Geometry: final body of the model. Coordinates: model frame, mm. Face numbers are marked on the shaded views. A direction names the side the tool comes from. Give positions to 0.01 mm unless a question says otherwise; leave off trailing zeros. Write each loop counter-clockwise with the first axis right and the second up, starting at its lowest first coordinate (ties: lowest second). Pieces come first, ordered by that corner, then holes. Notation, with made-up numbers: (-23.5, -27) -> (-19.5, -27) arc R25 cw to (-19.5, 5) -> close; hole circle Ø1 at (45, 17). An arc over 180 degrees is marked (long way). Answer in a Markdown table with one row per item. Add a question column.
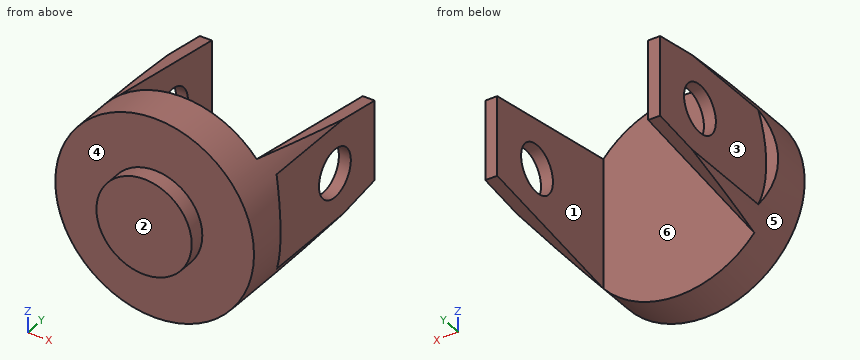
from build123d import *

# Parameters (mm, degrees)
SKETCH1_R               = 125
BOSS_EXTRUDE1_DEPTH     = 250
SKETCH3_W               = 190
SKETCH3_H               = 250
CUT_EXTRUDE1_DEPTH      = 200
CUT_EXTRUDE3_DEPTH      = 221
CUT_EXTRUDE3_DEPTH_BACK = 31
SKETCH8_R               = 30
CUT_EXTRUDE4_DEPTH      = 221
CUT_EXTRUDE4_DEPTH_BACK = 31
SKETCH6_R               = 125
CUT_EXTRUDE8_DEPTH      = 60
SKETCH7_R               = 125
CUT_EXTRUDE9_DEPTH      = 60
SKETCH9_R               = 59.95
BOSS_EXTRUDE2_DEPTH     = 20


with BuildPart() as part:
    # Sketch1 → Boss-Extrude1 (new body)
    with BuildSketch(Plane(origin=(0, 0, 0), x_dir=(1, 0, 0), z_dir=(0, 1, 0))):
        Circle(SKETCH1_R)
    extrude(amount=BOSS_EXTRUDE1_DEPTH)

    # Sketch3 → Cut-Extrude1 (cut)
    with BuildSketch(Plane(origin=(0, 250, 0), x_dir=(1, 0, 0), z_dir=(0, 1, 0))):
        Rectangle(SKETCH3_W, SKETCH3_H)
    extrude(amount=-CUT_EXTRUDE1_DEPTH, mode=Mode.SUBTRACT)

    # Sketch4 → Cut-Extrude3 (cut, two sides)
    with BuildSketch(Plane(origin=(-95, 0, 0), x_dir=(0, 0, -1), z_dir=(1, 0, 0))) as cut_extrude3_sk:
        Polygon((-81.240384046, 250), (-81.240384046, 50), (-50, 250), align=None)
        Polygon((50, 250), (81.240384046, 50), (81.240384046, 250), align=None)
    extrude(amount=CUT_EXTRUDE3_DEPTH, mode=Mode.SUBTRACT)
    extrude(cut_extrude3_sk.sketch, amount=-CUT_EXTRUDE3_DEPTH_BACK, mode=Mode.SUBTRACT)

    # Sketch8 → Cut-Extrude4 (cut, two sides)
    with BuildSketch(Plane(origin=(-95, 0, 0), x_dir=(0, 0, -1), z_dir=(1, 0, 0))) as cut_extrude4_sk:
        with Locations((0, 175)):
            Circle(SKETCH8_R)
    extrude(amount=CUT_EXTRUDE4_DEPTH, mode=Mode.SUBTRACT)
    extrude(cut_extrude4_sk.sketch, amount=-CUT_EXTRUDE4_DEPTH_BACK, mode=Mode.SUBTRACT)

    # Sketch6 → Cut-Extrude8 (cut)
    with BuildSketch(Plane(origin=(-170, 0, 0), x_dir=(0, 0, -1), z_dir=(1, 0, 0))):
        with Locations((0, 175)):
            Circle(SKETCH6_R)
    extrude(amount=CUT_EXTRUDE8_DEPTH, mode=Mode.SUBTRACT)

    # Sketch7 → Cut-Extrude9 (cut)
    with BuildSketch(Plane.ZY.offset(-170)):
        with Locations((0, 175)):
            Circle(SKETCH7_R)
    extrude(amount=CUT_EXTRUDE9_DEPTH, mode=Mode.SUBTRACT)

    # Sketch9 → Boss-Extrude2 (add)
    with BuildSketch(Plane.XZ):
        Circle(SKETCH9_R)
    extrude(amount=BOSS_EXTRUDE2_DEPTH)


solid = part.part
Q1. Line query: probe 1 along Y at (x, z) = (-103.5, 0); probe 2 along X at (y, z) = (146, -14); probe 3 along Y at (x, z) = (35.5, -78). Output: solid intervals per line, ascending. Write a range as from..to.
Q2. Section A-A on z = 0. Return loops of the section in (x, y), and give its area (3 significant figures).
Q3. Section C-C on x = 0. Return loops of the section in (y, z), and give its area (3 significant figures).
Q4. Access query for the marked faces 4, 5 and 6. Directions: +Z, -Z, +X, -X, +Y, -Y. A direction counts if a zero-diameter tool reaches every point of the face in a straight line with its end or side. Return the directions, or none.
Q5. Pull-direction query (X, two-part tool) for the marked faces 1, 2 and 3; classes: +X half, -X half, draft (parallel to the pull), parting line (faces both ways), or undercut.
Q6. Contact query for flat-ended pins moving along their axis: pin 1 Ø1.5 at (x, z) = (87.5, -36.5) entering from +Y; pin 2 Ø6 at (y, z) = (78.5, 43.5) entering from +X; pin 3 Ø12 at (x, y) = (-50, 8.5) entering from -Z. Output: stop coordinate, or through.
Q7. Section D-D on y = 175. Return loops of the section in (x, z).
Q8. Section B-B on y = 117. Return loops of the section in (x, z).
Checks:
| question | item | result |
|---|---|---|
| 1 | probe 1 | 0..145, 205..250 |
| 1 | probe 2 | -110..-95, 95..110 |
| 1 | probe 3 | 0..50 |
| 2 | outline | (-125, 0) -> (-59.95, 0) -> (-59.95, -20) -> (59.95, -20) -> (59.95, 0) -> (125, 0) -> (125, 50) -> (110, 50) -> (110, 145) -> (95, 145) -> (95, 50) -> (-95, 50) -> (-95, 145) -> (-110, 145) -> (-110, 50) -> (-125, 50) -> close; (-110, 205) -> (-95, 205) -> (-95, 250) -> (-110, 250) -> close; (95, 205) -> (110, 205) -> (110, 250) -> (95, 250) -> close |
| 2 | area | 19,100 mm^2 |
| 3 | outline | (-20, -59.95) -> (0, -59.95) -> (0, -125) -> (50, -125) -> (50, 125) -> (0, 125) -> (0, 59.95) -> (-20, 59.95) -> close |
| 3 | area | 14,900 mm^2 |
| 4 | face 4 | -Y |
| 4 | face 5 | +Y, -Y |
| 4 | face 6 | +Z, -Z, +Y |
| 5 | face 1 | undercut |
| 5 | face 2 | draft |
| 5 | face 3 | -X half |
| 6 | pin 1 | y = 50 |
| 6 | pin 2 | x = 110 |
| 6 | pin 3 | z = -117 |
| 7 | outline | (-110, -59.37) arc R125 ccw to (-108.7, -61.72) -> (-95, -61.72) -> (-95, -30) -> (-110, -30) -> close; (-110, 30) -> (-95, 30) -> (-95, 61.72) -> (-108.7, 61.72) arc R125 ccw to (-110, 59.37) -> close; (95, -61.72) -> (108.7, -61.72) arc R125 ccw to (110, -59.37) -> (110, -30) -> (95, -30) -> close; (95, 30) -> (110, 30) -> (110, 59.37) arc R125 ccw to (108.7, 61.72) -> (95, 61.72) -> close |
| 8 | outline | (-110, -59.37) arc R125 ccw to (-103.03, -70.77) -> (-95, -70.77) -> (-95, 70.77) -> (-103.03, 70.77) arc R125 ccw to (-110, 59.37) -> close; (95, -70.77) -> (103.03, -70.77) arc R125 ccw to (110, -59.37) -> (110, 59.37) arc R125 ccw to (103.03, 70.77) -> (95, 70.77) -> close |
